from build123d import *

# Parameters (mm, degrees)
SALIENTE_EXTRUIR1_DEPTH = 39.5
CROQUIS2_R              = 11
CROQUIS2_R_2            = 3.75
SALIENTE_EXTRUIR2_DEPTH = 2
CROQUIS3_R              = 16.25
CROQUIS3_R_2            = 11
CORTAR_EXTRUIR2_DEPTH   = 0.5
CROQUIS4_R              = 2.75
EJE_DEPTH               = 42.5
CROQUIS5_R              = 3.5
PERNOSATRAS_DEPTH       = 2
CROQUIS6_R              = 1.5
PERNOSFRENTE_DEPTH      = 5
CROQUIS7_R              = 2.75
SALIENTE_EXTRUIR3_DEPTH = 55
CROQUIS8_R              = 6.75
SALIENTE_EXTRUIR4_DEPTH = 7


with BuildPart() as part:
    # Croquis1 → Saliente-Extruir1 (new body)
    with BuildSketch(Plane(origin=(0, 0, 0), x_dir=(1, 0, 0), z_dir=(0, 1, 0))):
        Polygon((-16.6, 21.1), (-21.1, 16.6), (-21.1, -16.6), (-16.6, -21.1), (16.6, -21.1), (21.1, -16.6), (21.1, 16.6), (16.6, 21.1), align=None)
    extrude(amount=SALIENTE_EXTRUIR1_DEPTH)

    # Croquis2 → Saliente-Extruir2 (add)
    with BuildSketch(Plane(origin=(0, 39.5, 0), x_dir=(1, 0, 0), z_dir=(0, 1, 0))):
        Circle(CROQUIS2_R)
        Circle(CROQUIS2_R_2, mode=Mode.SUBTRACT)
    extrude(amount=SALIENTE_EXTRUIR2_DEPTH)

    # Croquis3 → Cortar-Extruir2 (cut)
    with BuildSketch(Plane(origin=(0, 39.5, 0), x_dir=(1, 0, 0), z_dir=(0, 1, 0))):
        Circle(CROQUIS3_R)
        Circle(CROQUIS3_R_2, mode=Mode.SUBTRACT)
    extrude(amount=-CORTAR_EXTRUIR2_DEPTH, mode=Mode.SUBTRACT)

    # Croquis4 → EJE (cut, through all)
    with BuildSketch(Plane(origin=(0, 41.5, 0), x_dir=(1, 0, 0), z_dir=(0, 1, 0))):
        Circle(CROQUIS4_R)
    extrude(amount=-EJE_DEPTH, mode=Mode.SUBTRACT)

    # Croquis5 → PernosAtras (cut)
    with BuildSketch(Plane.XZ):
        with Locations((-15.6, 15.6)):
            Circle(CROQUIS5_R)
        with Locations((15.6, 15.6)):
            Circle(CROQUIS5_R)
        with Locations((15.6, -15.6)):
            Circle(CROQUIS5_R)
        with Locations((-15.6, -15.6)):
            Circle(CROQUIS5_R)
    extrude(amount=-PERNOSATRAS_DEPTH, mode=Mode.SUBTRACT)

    # Croquis6 → PernosFrente (cut)
    with BuildSketch(Plane(origin=(0, 39.5, 0), x_dir=(1, 0, 0), z_dir=(0, 1, 0))):
        with Locations((-15.6, 15.6)):
            Circle(CROQUIS6_R)
        with Locations((15.6, 15.6)):
            Circle(CROQUIS6_R)
        with Locations((15.6, -15.6)):
            Circle(CROQUIS6_R)
        with Locations((-15.6, -15.6)):
            Circle(CROQUIS6_R)
    extrude(amount=-PERNOSFRENTE_DEPTH, mode=Mode.SUBTRACT)

    # Croquis7 → Saliente-Extruir3 (add)
    with BuildSketch(Plane.XZ):
        Circle(CROQUIS7_R)
    extrude(amount=-SALIENTE_EXTRUIR3_DEPTH)

    # Croquis8 → Saliente-Extruir4 (add)
    with BuildSketch(Plane(origin=(0, 55, 0), x_dir=(1, 0, 0), z_dir=(0, 1, 0))):
        Circle(CROQUIS8_R)
    extrude(amount=-SALIENTE_EXTRUIR4_DEPTH)


solid = part.part
Design review of the part built by this model. Coordinates are the model's own, in mm. A direction names the side the tool comes from. Coordinates: 2 decimals unless noted, no trailing zeros. Order: outer loops, then holes, each group sorted by start corner. A loop starts at its lowest first (then second) coordinate and runs counter-clockwise, first axis right, second up.
Item 1: Take a section at C-C, the plane z = 6. Write out the cut boundary in (x, y), then the cut area to 3 significant figures.
Item 2: The part is to be moulded in two halves that separate along Z. For faces 5 (the flat face through (-16, 34.5, -16)), 6 (the flat face through (-16, 34.5, 16)), 7 (the flat face through (9, 39.5, 14)), 8 (the cylindrical face through (-1.46, 51.55, 6.59)), say which applies: pulls with the +Z half, pulls with the -Z half, needs draft (parallel to the pull), parting line crosses it, or undercut.
Item 3: Take a section at D-D, the plane y = 23. Write out the cut boundary in (x, z), then the cut area to 3 significant figures.
Item 4: For faces 1 (the cylindrical face through (-16.71, 37.03, 14.59)), 2 (the flat face through (3, 48, 0)), 3 (the flat face through (-21.1, 19, 0)), 4 (the flat face through (16, 2, 16)), list the 3-axis set-ups (+Z, -Z, +X, -X, +Y, -Y) from which the entire face can be reached by the end or side of a thin tool; tool diameter is ignored.
Item 5: Take a section at B-B, the plane x = 15.6. Write out the cut boundary in (y, z), then the cut area to 3 significant figures.
Item 6: For line 1 (Z direction, x = 0, y = 39.4); line 2 (Z direction, x = -15.6, y = 1.5); line 3 (X direction, y = 40, z = 0), list the stretches that pass through material, from the lowest coordinate up.
Item 7: For pin 1 Ø0.9 at (x, z) = (-16, -15.5) entering from +Y; pin 2 Ø12 at (x, z) = (-11.5, -10) entering from +Y; pin 3 Ø4 at (x, y) = (9, 42) entering from -Z, all flat-tipped, find the tip position at first contact; note any pin that passes through.
Item 8: Take a section at A-A, the plane x = -6. Write out the cut boundary in (y, z), then the cut area to 3 significant figures.
The answers:
1. outline: (-21.1, 0) - (21.1, 0) - (21.1, 39.5) - (15.1, 39.5) - (15.1, 39) - (9.22, 39) - (9.22, 41.5) - (-9.22, 41.5) - (-9.22, 39) - (-15.1, 39) - (-15.1, 39.5) - (-21.1, 39.5) - close; (-3.09, 48) - (3.09, 48) - (3.09, 55) - (-3.09, 55) - close
1. area: 1,740 mm2
2. face 5: undercut
2. face 6: undercut
2. face 7: needs draft
2. face 8: parting line crosses it
3. outline: (-21.1, -16.6) - (-16.6, -21.1) - (16.6, -21.1) - (21.1, -16.6) - (21.1, 16.6) - (16.6, 21.1) - (-16.6, 21.1) - (-21.1, 16.6) - close
3. area: 1,740 mm2
4. face 1: +Y
4. face 2: none
4. face 3: +Z, -Z, -X, +Y, -Y
4. face 4: -Y
5. outline: (0, -21.1) - (39.5, -21.1) - (39.5, -17.1) - (34.5, -17.1) - (34.5, -14.1) - (39.5, -14.1) - (39.5, -4.55) - (39, -4.55) - (39, 4.55) - (39.5, 4.55) - (39.5, 14.1) - (34.5, 14.1) - (34.5, 17.1) - (39.5, 17.1) - (39.5, 21.1) - (0, 21.1) - (0, 19.1) - (2, 19.1) - (2, 12.1) - (0, 12.1) - (0, -12.1) - (2, -12.1) - (2, -19.1) - (0, -19.1) - close
5. area: 1,600 mm2
6. line 1: z = -21.1 to -16.25, -11 to 11, 16.25 to 21.1
6. line 2: z = -21.1 to -19.1, -12.1 to 12.1, 19.1 to 21.1
6. line 3: x = -11 to -3.75, -2.75 to 2.75, 3.75 to 11
7. pin 1: stops at y = 34.5
7. pin 2: stops at y = 41.5
7. pin 3: stops at z = -8.43
8. outline: (0, -21.1) - (39.5, -21.1) - (39.5, -15.1) - (39, -15.1) - (39, -9.22) - (41.5, -9.22) - (41.5, 9.22) - (39, 9.22) - (39, 15.1) - (39.5, 15.1) - (39.5, 21.1) - (0, 21.1) - close; (48, -3.09) - (55, -3.09) - (55, 3.09) - (48, 3.09) - close
8. area: 1,740 mm2
